Here's how the part is built. I have some questions about the finished solid (model axes, mm). A direction names the side the tool comes from. Round coordinates to 2 decimals unless told otherwise and drop trailing zeros. Loops run counter-clockwise (first coordinate to the right, second up) from the corner with the lowest first, then second, coordinate; pieces in that order, holes last. Notation, with made-up numbers: (-22, 88.5) - (8, 88.5) arc R17 cw to (8, 121.5) - close; hole circle Ø6 at (3.25, 27.25). An arc over 180 degrees is marked (long way). Return JSON: item names as keys, results as strings. Group by question number.
```python
from build123d import *

# Parameters (mm, degrees)
BOSS_EXTRUDE1_START = 20
SKETCH1_R           = 40
BOSS_EXTRUDE1_DEPTH = 120
CUT_EXTRUDE1_START  = 20
SKETCH1_4_R         = 25
CUT_EXTRUDE1_DEPTH  = 40
SKETCH2_R           = 7.5
SKETCH2_W           = 36.544112996
SKETCH2_H           = 10
CUT_EXTRUDE2_DEPTH  = 262.537261524


with BuildPart() as part:
    # Sketch1 → Boss-Extrude1 (new body)
    with BuildSketch(Plane(origin=(0, 0, 0), x_dir=(1, 0, 0), z_dir=(0, 1, 0)).offset(BOSS_EXTRUDE1_START)):
        with Locations(Location((131.582372263, -99.144632286, 0), (0, 0, 270))):
            Circle(SKETCH1_R)
    extrude(amount=BOSS_EXTRUDE1_DEPTH)

    # Sketch1<4> → Cut-Extrude1 (cut)
    with BuildSketch(Plane(origin=(0, 0, 0), x_dir=(1, 0, 0), z_dir=(0, 1, 0)).offset(CUT_EXTRUDE1_START)):
        with Locations(Location((131.582372263, -99.144632286, 0), (0, 0, 270))):
            Circle(SKETCH1_4_R)
    extrude(amount=CUT_EXTRUDE1_DEPTH, mode=Mode.SUBTRACT)

    # Sketch2 → Cut-Extrude2 (cut, through all)
    with BuildSketch(Plane.XY):
        with Locations(Location((116.582372263, 90, 0), (0, 0, 180))):
            Circle(SKETCH2_R)
        Polygon((113.167198818, 142), (173.582372263, 70), (173.582372263, 142), align=None)
        with Locations((107.854428761, 120)):
            Rectangle(SKETCH2_W, SKETCH2_H)
    extrude(amount=CUT_EXTRUDE2_DEPTH, mode=Mode.SUBTRACT)


solid = part.part
```
Q1. If we mould it in two halves opening along Y, with no side actions, what happens to faces 1 (the cylindrical face through (156.37, 39.72, 95.89)), 2 (the flat face through (106, 140, 99)), 3 (the cylindrical face through (124.075, 89.67, 98.595))? For each: +Y half, -Y half, draft (parallel to the pull), parting line (faces both ways), or undercut.
Q2. Will these pins go through, and if not, where does the flat tip stop? pin 1 Ø6 at (x, y) = (110.5, 123.5) entering from +Z; pin 2 Ø1 at (x, z) = (162, 89) entering from +Y; pin 3 Ø5 at (x, y) = (150.5, 92.5) entering from +Z.
Q3. Imagine slicing it at B-B, the plane z = 76. List the corners of the cut face in (x, y) for me.
Q4. Imagine slicing it at A-A, the plane x = 103. List the corners of the cut face in (y, z) for me, and give its area (3 significant figures).
Q5. Please list where these lines run through material, in increasing order: line 1 (Y direction, x = 97.5, z = 112.5); line 2 (Y direction, x = 113.5, z = 131.5); line 3 (X direction, y = 96, z = 126).
Q6. For faces 4 (the cylindrical face through (92.534, 65.827, 90.473)), 5 (the flat face through (132, 60, 99)), 6 (the flat face through (112, 115, 99)), which set-ups out of +Z, -Z, +X, -X, +Y, -Y let a thin tool reach every point of the face, with its end or its side?
Q7. Imagine slicing it at D-D, the plane x = 142.5. List the corners of the cut face in (y, z) for me, and give its area (3 significant figures).
Q8. Imagine slicing it at C-C, the plane y = 90. List the corners of the cut face in (x, z) for me.
Output values:
{
 "1": {"face 1": "draft", "face 2": "+Y half", "face 3": "undercut"},
 "2": {"pin 1": "stops at z = 134.62", "pin 2": "stops at y = 84.4", "pin 3": "stops at z = 135.62"},
 "3": {"outline": "(98.96, 20) - (122.13, 20) - (122.13, 60) - (141.03, 60) - (141.03, 20) - (164.21, 20) - (164.21, 81.17) - (114.85, 140) - (98.96, 140) - (98.96, 125) - (126.13, 125) - (126.13, 115) - (98.96, 115) - close; hole circle Ø15 at (116.58, 90)"},
 "4": {"outline": "(20, 71.16) - (115, 71.16) - (115, 127.13) - (20, 127.13) - close; (125, 71.16) - (140, 71.16) - (140, 127.13) - (125, 127.13) - close", "area": "6,160 mm^2"},
 "5": {"line 1": "y = 20 to 115, 125 to 140", "line 2": "y = 20 to 83.16, 96.84 to 115, 125 to 140", "line 3": "x = 101.94 to 112.08, 121.08 to 151.77"},
 "6": {"face 4": "+Y, -Y", "face 5": "-Y", "face 6": "+Z, -Z, -X"},
 "7": {"outline": "(20, 60.66) - (107.04, 60.66) - (107.04, 137.63) - (20, 137.63) - (20, 121.63) - (60, 121.63) - (60, 76.65) - (20, 76.65) - close", "area": "4,900 mm^2"},
 "8": {"outline": "(109.08, 66.07) - (109.08, 132.22) arc R40 ccw to start; (124.08, 59.85) arc R40 ccw to (156.8, 68.1) - (156.8, 130.19) arc R40 ccw to (124.08, 138.44) - close"}
}
